Part model, mm, in its own coordinate system. A direction names the side the tool comes from. Coordinates: 2 decimals unless noted, no trailing zeros. Write each loop counter-clockwise with the first axis right and the second up, starting at its lowest first coordinate (ties: lowest second). Pieces come first, ordered by that corner, then holes. Notation, with made-up numbers: M 75,58 L 110,58 A13 cw 110,73 Z; hole C 35,81.25 d11. An arc over 180 degrees is marked long. Use a Markdown table: item, result. Add a question column.
Q1. Slice it at A-A on x = 0. Write the cut outline in (y, z), then the cut area to 3 significant figures.
Q2. Wall check: L1, parallel to X at y = 133, z = -0.25; L2, parallel to Y at x = 0, z = 3.25; L3, parallel to Z at x = 30, y = 11.75. Give the ranges that are in metal, low to high. Write a range as from..to.
Q3. Mould opens along Y. For faces 1 (the cylindrical face through (15.594, 97.719, -9.014)), 2 (the flat face through (-30, 110, 0)), 3 (the flat face through (28, 135, 0)) say: released by +Y, released by -Y, zero draft, split by the parting line, or undercut.
Q4. Tool access for faces 4 (the cylindrical face through (-15.719, 97.594, -9.014)), 5 (the cylindrical face through (-24.26, 50.73, 6.6)), 6 (the flat face through (20, 74, -10)), 7 (the flat face through (22, 137, 0)), 8 (the flat face through (-28, 135, 0)): list every direction of +Z, -Z, +X, -X, +Y, -Y with a clear straight run to the whole face (end or side of a thin tool).
Q5. Pin check, flat tips, straight feed: pin 1 Ø17 at (x, y) = (-12, 56.5) entering from -Z; pin 2 Ø1.6 at (y, z) = (88, -9) entering from -X; pin 3 Ø10 at (x, y) = (0.5, 42) entering from +Z; pin 4 Ø1 at (x, z) = (19, -5.5) entering from -Y. Stop position of each tip, or through.
from build123d import *

# Parameters (mm, degrees)
SKETCH1_R                         = 6.5
BOSS_EXTRUDE1_DEPTH               = 10
SKETCH2_R                         = 10
CUT_EXTRUDE1_DEPTH                = 14
CHAMFER1_SIZE                     = 1
CHAMFER2_SIZE                     = 4
FILLET1_R                         = 5
CUT_EXTRUDE2_DEPTH                = 4
FILLET2_R                         = 2
FILLET2_OF_MIRROR2_R              = 2
M10X1_25_TAPPED_HOLE1_D           = 8.8
M10X1_25_TAPPED_HOLE1_DEPTH       = 20
M10X1_25_TAPPED_HOLE1_CSINK_D     = 10.05
M10X1_25_TAPPED_HOLE1_CSINK_ANGLE = 90
M10X1_25_TAPPED_HOLE1_TIP         = 2.643786724


with BuildPart() as part:
    # Sketch1 → Boss-Extrude1 (new, symmetric)
    with BuildSketch(Plane.XY):
        with BuildLine():
            Line((-46, 0), (46, 0))
            Line((46, 0), (46, 15))
            Line((46, 15), (31.449256053, 74.112397284))
            ThreePointArc((31.449256053, 74.112397284), (30.363636327, 80.044097084), (30, 86.06334964))
            Line((30, 86.06334964), (30, 137))
            Line((30, 137), (16, 137))
            ThreePointArc((16, 137), (0, 145), (-16, 137))
            Line((-16, 137), (-30, 137))
            Line((-30, 137), (-30, 86.06334964))
            ThreePointArc((-30, 86.06334964), (-30.363636327, 80.044097084), (-31.449256053, 74.112397284))
            Line((-31.449256053, 74.112397284), (-46, 15))
            Line((-46, 15), (-46, 0))
        make_face()
        with Locations((0, 125)):
            Circle(SKETCH1_R, mode=Mode.SUBTRACT)
    extrude(amount=BOSS_EXTRUDE1_DEPTH, both=True)

    # Sketch2 → Cut-Extrude1 (cut)
    with BuildSketch(Plane.XY.offset(10)):
        with Locations((0, 125)):
            Circle(SKETCH2_R)
    extrude(amount=-CUT_EXTRUDE1_DEPTH, mode=Mode.SUBTRACT)

    # Chamfer1
    chamfer1_edges = [part.edges().sort_by_distance(p)[0] for p in [
        (-10, 125, 10),
    ]]
    chamfer(chamfer1_edges, length=CHAMFER1_SIZE)

    # Chamfer2
    chamfer2_edges = [part.edges().sort_by_distance(p)[0] for p in [
        (-30, 137, 0),
        (30, 137, 0),
    ]]
    chamfer(chamfer2_edges, length=CHAMFER2_SIZE)

    # Fillet1
    fillet1_edges = [part.edges().sort_by_distance(p)[0] for p in [
        (-16, 137, 0),
        (16, 137, 0),
    ]]
    fillet(fillet1_edges, radius=FILLET1_R)

    # Sketch10 → Cut-Extrude2 (cut)
    with BuildSketch(Plane.XY.offset(10)):
        with BuildLine():
            ThreePointArc((18, 86.06334964), (18.450909046, 78.59947647), (19.797077506, 71.244168718))
            Line((19.797077506, 71.244168718), (29.971112298, 29.912152377))
            ThreePointArc((29.971112298, 29.912152377), (28.49970745, 23.065287193), (22.202993266, 20))
            Line((22.202993266, 20), (-22.202993266, 20))
            ThreePointArc((-22.202993266, 20), (-28.49970745, 23.065287193), (-29.971112298, 29.912152377))
            Line((-29.971112298, 29.912152377), (-19.797077506, 71.244168718))
            ThreePointArc((-19.797077506, 71.244168718), (-18.450909046, 78.59947647), (-18, 86.06334964))
            Line((-18, 86.06334964), (-18, 92))
            ThreePointArc((-18, 92), (-15.656854249, 97.656854249), (-10, 100))
            Line((-10, 100), (10, 100))
            ThreePointArc((10, 100), (15.656854249, 97.656854249), (18, 92))
            Line((18, 92), (18, 86.06334964))
        make_face()
    cut_extrude2 = extrude(amount=-CUT_EXTRUDE2_DEPTH, mode=Mode.SUBTRACT)

    # Fillet2
    fillet2_edges = [part.edges().sort_by_distance(p)[0] for p in [
        (-24.884094902, 50.578160548, 6),
        (-18, 89.03167482, 6),
        (15.656854249, 97.656854249, 6),
        (18, 89.03167482, 6),
        (18.450909046, 78.59947647, 6),
        (-28.49970745, 23.065287193, 6),
        (-18.450909046, 78.59947647, 6),
        (-15.656854249, 97.656854249, 6),
        (0, 100, 6),
        (24.884094902, 50.578160548, 6),
        (28.49970745, 23.065287193, 6),
        (0, 20, 6),
    ]]
    fillet(fillet2_edges, radius=FILLET2_R)

    # Mirror2: Cut-Extrude2 across plane
    add(cut_extrude2.mirror(Plane.XY), mode=Mode.SUBTRACT)

    # Fillet2 of Mirror2
    fillet2_of_mirror2_edges = [part.edges().sort_by_distance(p)[0] for p in [
        (-24.884094902, 50.578160548, -6),
        (-18, 89.03167482, -6),
        (15.656854249, 97.656854249, -6),
        (18, 89.03167482, -6),
        (18.450909046, 78.59947647, -6),
        (-28.49970745, 23.065287193, -6),
        (-18.450909046, 78.59947647, -6),
        (-15.656854249, 97.656854249, -6),
        (0, 100, -6),
        (24.884094902, 50.578160548, -6),
        (28.49970745, 23.065287193, -6),
        (0, 20, -6),
    ]]
    fillet(fillet2_of_mirror2_edges, radius=FILLET2_OF_MIRROR2_R)

    # M10x1.25 Tapped Hole1
    with Locations(Plane(origin=(0, 0, 0), x_dir=(-1, 0, 0), z_dir=(0, -1, 0))):
        with Locations((-30, 0), (30, 0)):
            CounterSinkHole(M10X1_25_TAPPED_HOLE1_D / 2, M10X1_25_TAPPED_HOLE1_CSINK_D / 2, depth=M10X1_25_TAPPED_HOLE1_DEPTH, counter_sink_angle=M10X1_25_TAPPED_HOLE1_CSINK_ANGLE)
            with Locations((0, 0, -(M10X1_25_TAPPED_HOLE1_DEPTH + M10X1_25_TAPPED_HOLE1_TIP / 2))):  # 118° drill point
                Cone(0, M10X1_25_TAPPED_HOLE1_D / 2, M10X1_25_TAPPED_HOLE1_TIP, mode=Mode.SUBTRACT)


solid = part.part
Recorded:
| question | item | result |
|---|---|---|
| 1 | outline | M 0,-10 L 20,-10 L 20,-8 A2 cw 22,-6 L 98,-6 A2 cw 100,-8 L 100,-10 L 118.5,-10 L 118.5,-4 L 115,-4 L 115,9 L 114,10 L 100,10 L 100,8 A2 cw 98,6 L 22,6 A2 cw 20,8 L 20,10 L 0,10 Z; M 131.5,-10 L 145,-10 L 145,10 L 136,10 L 135,9 L 135,-4 L 131.5,-4 Z |
| 1 | area | 1,900 mm² |
| 2 | L1 | -30..-6, 6..30 |
| 2 | L2 | 0..115, 135..145 |
| 2 | L3 | -10..-4.4, 4.4..10 |
| 3 | face 1 | undercut |
| 3 | face 2 | zero draft |
| 3 | face 3 | released by +Y |
| 4 | face 4 | -Z |
| 4 | face 5 | +Z |
| 4 | face 6 | -Z, +X, -X, +Y, -Y |
| 4 | face 7 | +Z, -Z, +X, +Y |
| 4 | face 8 | +Z, -Z, -X, +Y |
| 5 | pin 1 | z = -6 |
| 5 | pin 2 | x = -30 |
| 5 | pin 3 | z = 6 |
| 5 | pin 4 | y = 0 |
